Autodesk Inventor part; units mm, degrees
ref_plane "YZ Plane" through (0, 0, 0) normal (1, 0, 0) x (0, 1, 0)
ref_plane "XZ Plane" through (0, 0, 0) normal (0, 1, 0) x (-1, 0, 0)
ref_plane "XY Plane" through (0, 0, 0) normal (0, 0, 1) x (1, 0, 0)
sketch "Sketch1" plane through (0, 0, 0) normal (0, 1, 0) x (-1, 0, 0)
  line L0 (0, 0) -> (0, -0.5031)
  line L1 (9.8697, 13.5923) -> (193.7822, 80.5309)
  line L2 (166.1465, 0) -> (0, 0) construction
  line L3 (0, 0) -> (0, 0.5031)
  line L4 (9.8697, -13.5923) -> (193.7822, -80.5309)
  circle A0 centre (50, 0) radius 12.5
  circle A1 centre (63.5, 13.5) radius 1.5
  circle A2 centre (63.5, -13.5) radius 1.5
  circle A3 centre (36.5, 13.5) radius 1.5
  circle A4 centre (36.5, -13.5) radius 1.5
  line L5 (63.5, 13.5) -> (36.5, -13.5) construction
  line L6 (36.5, 13.5) -> (63.5, -13.5) construction
  arc A5 (9.8697, 13.5923) -> (0, -0.5031) centre (15, -0.5031) ccw
  arc A6 (0, 0.5031) -> (9.8697, -13.5923) centre (15, 0.5031) ccw
  line L7 (63.25, 16.25) -> (36.75, 16.25)
  line L8 (33.75, 13.25) -> (33.75, -13.25)
  line L9 (36.75, -16.25) -> (63.25, -16.25)
  line L10 (66.25, -13.25) -> (66.25, 13.25)
  line L11 (66.25, 16.25) -> (33.75, -16.25) construction
  line L12 (33.75, 16.25) -> (66.25, -16.25) construction
  arc A7 (66.25, 13.25) -> (63.25, 16.25) centre (63.25, 13.25) ccw
  arc A8 (63.25, -16.25) -> (66.25, -13.25) centre (63.25, -13.25) ccw
  arc A9 (33.75, -13.25) -> (36.75, -16.25) centre (36.75, -13.25) ccw
  arc A10 (36.75, 16.25) -> (33.75, 13.25) centre (36.75, 13.25) ccw
  line L13 (197.8082, 77.7119) -> (197.8082, -77.7119)
  line L14 (190.7822, 76.2465) -> (10.8958, 10.7732)
  arc A11 (10.8958, 10.7732) -> (3, -0.5031) centre (15, -0.5031) ccw
  line L15 (3, -0.5031) -> (3, 0)
  line L16 (3, 0) -> (3, 0.5031)
  arc A12 (3, 0.5031) -> (10.8958, -10.7732) centre (15, 0.5031) ccw
  line L17 (10.8958, -10.7732) -> (190.7822, -76.2465)
  line L18 (194.8082, -73.4274) -> (194.8082, 73.4274)
  arc A13 (197.8082, 77.7119) -> (193.7822, 80.5309) centre (194.8082, 77.7119) ccw
  arc A14 (194.8082, 73.4274) -> (190.7822, 76.2465) centre (191.8082, 73.4274) ccw
  arc A15 (190.7822, -76.2465) -> (194.8082, -73.4274) centre (191.8082, -73.4274) ccw
  arc A16 (193.7822, -80.5309) -> (197.8082, -77.7119) centre (194.8082, -77.7119) ccw
  point P0 (0, 10)
  point P1 (197.8082, 81.9963)
  point P2 (0, -10)
  point P3 (197.8082, -81.9963)
  point P4 (50, 0)
  point P5 (194.8082, 77.7119)
  point P6 (194.8082, -77.7119)
  point P7 (0.0084, 0)
  point P8 (3.0106, 0)
  dimension "d1" = 25
  dimension "d2" = 50
  dimension "d3" = 27
  dimension "d4" = 27
  dimension "d5" = 3
  dimension "d6" = 15
  dimension "d7" = 10
  dimension "d9" = 70
  dimension "d10" = 32.5
  dimension "d11" = 3
  dimension "d12" = 200
  dimension "d13" = 3
  dimension "d20" = 3
extrude "Extrusion1" add sketch "Sketch1" along normal blind 2 contours A5 L1 A13 L13 A16 L4 A6 | A0 | A1 | A2 | A3 | A4 | A7 L10 A8 L9 A9 L8 A10 L7 | A14 L18 A15 L17 A12 A11 L14 | A11 L15 L16 A12
extrude "Extrusion2" cut sketch "Sketch1" along normal blind 2 contours A0 | A1 | A2 | A3 | A4
properties part number "PRTGN_baseipt"
Here's how the part is built. I have some questions about the finished solid (model axes, mm). Give positions to 0.01 mm unless a question says otherwise; leave off trailing zeros. Write each loop counter-clockwise with the first axis right and the second up, starting at its lowest first coordinate (ties: lowest second). Pieces come first, ordered by that corner, then holes. Notation, with made-up numbers: (36, 25.25) -> (50, 25.25) arc R16 ccw to (50, 49.25) -> close; hole circle Ø5 at (45, -35). An arc over 180 degrees is marked (long way). Use one line per item in the form item = value.
1) We'd pull the mould along Z, two halves only. Please class faces 1 (the face through (-100.539, 0.986, 46.593)), 2 (the face through (-120, 0, 1)), 3 (the face through (-37.512, 0.986, -0.55)), 4 (the face through (-100.539, 0.986, -46.593)): +Z half, -Z half, draft (parallel to the pull), parting line (faces both ways), or undercut.
Verdict:
face_1 = +Z half
face_2 = draft
face_3 = undercut
face_4 = -Z half
2) Suppose I cut it at D-D (x = -133.5). Please give me the cut outline in (y, z), and give its area (3 significant figures).
Verdict:
outline = (0, -58.59) -> (2, -58.59) -> (2, 58.59) -> (0, 58.59) -> close
area = 234 mm2
3) Suppose I cut it at C-C (x = -50). Please give me the cut outline in (y, z).
Verdict:
outline = (0, -28.2) -> (2, -28.2) -> (2, -12.5) -> (0, -12.5) -> close; (0, 12.5) -> (2, 12.5) -> (2, 28.2) -> (0, 28.2) -> close
4) Suppose I cut it at B-B (z = -9). Please give me the cut outline in (x, y), and give its area (3 significant figures).
Verdict:
outline = (-197.81, 0) -> (-58.67, 0) -> (-58.67, 2) -> (-197.81, 2) -> close; (-41.33, 0) -> (-3.39, 0) -> (-3.39, 2) -> (-41.33, 2) -> close
area = 354 mm2
5) I'm going to push flat-ended pins straight in: pin 1 (2.5 mm diameter, centred on x = -63.5, z = 13.5, fed in from +Y); pin 2 (3.5 mm diameter, centred on x = -36.5, z = -13.5, fed in from -Y); pin 3 (1 mm diameter, centred on x = -145.5, y = 0.5, fed in from -Z). Where does each tip first touch, or does it pass through?
Verdict:
pin_1 = through
pin_2 = 0
pin_3 = -63.14
6) If I drill on L1, parallel to Z at x = -63.5, y = 1.3; L2, parallel to Z at x = -36.5, y = 0.5; L3, parallel to X at y = 0.4, z = -3, over which ranges is the centre line in solid material (lowest first)? Write a range as [from, to].
Verdict:
L1 = [-33.11, -15], [-12, 12], [15, 33.11]
L2 = [-23.28, -15], [-12, 12], [15, 23.28]
L3 = [-197.81, -62.13], [-37.87, -0.41]
7) Suppose I cut it at A-A (y = 0.95). Please give me the cut outline in (x, z), and give its area (3 significant figures).
Verdict:
outline = (-197.81, -77.71) arc R3 ccw to (-193.78, -80.53) -> (-9.87, -13.59) arc R15 ccw to (-0.01, 0) arc R15 ccw to (-9.87, 13.59) -> (-193.78, 80.53) arc R3 ccw to (-197.81, 77.71) -> close; hole circle Ø3 at (-63.5, -13.5); hole circle Ø3 at (-63.5, 13.5); hole circle Ø25 at (-50, 0); hole circle Ø3 at (-36.5, -13.5); hole circle Ø3 at (-36.5, 13.5)
area = 17,600 mm2
